```python
from build123d import *

# Parameters (mm, degrees)
PAD_DEPTH          = 38
POCKET_DEPTH       = 32
SKETCH002_R        = 6.25
POCKET001_DEPTH    = 6
CHAMFER_SIZE       = 1
SKETCH003_R        = 1.6
SKETCH003_R_2      = 3
POCKET002_DEPTH    = 7
SKETCH004_R        = 6.5
POCKET003_DEPTH    = 3
SKETCH005_R        = 1.45
POCKET004_DEPTH    = 5
POLARPATTERN_COUNT = 6
SKETCH006_R        = 3
SKETCH006_R_2      = 1.6
PAD001_DEPTH       = 1.5


with BuildPart() as part:
    # Sketch → Pad (new body)
    with BuildSketch(Plane.XY):
        with BuildLine():
            ThreePointArc((-41.5784274686, 27.7711067341), (32.1393804843, -38.3022221559), (-20.1291830613, 45.7691598053))
            Line((-41.5784274686, 27.7711067341), (-20.1291830613, 45.7691598053))
        make_face()
    extrude(amount=PAD_DEPTH)

    # Sketch001 → Pocket (cut)
    with BuildSketch(Plane.XY.offset(38)):
        with BuildLine():
            ThreePointArc((-41.314902238, 15.1353511047), (28.2826548262, -33.7059554972), (-7.7311536284, 43.3154621766))
            Line((-21.2649980047, 40.8998760372), (-7.7311536284, 43.3154621766))
            Line((-36.5858868671, 28.0441238435), (-21.2649980047, 40.8998760372))
            Line((-36.5858868671, 28.0441238435), (-41.314902238, 15.1353511047))
        make_face()
    extrude(amount=-POCKET_DEPTH, mode=Mode.SUBTRACT)

    # Sketch002 (on Face2 of Pocket) → Pocket001 (cut)
    with BuildSketch(Plane(origin=(-30.853805265, 36.7701332697, 0), x_dir=(-0.7660444431, -0.6427876097, 0), z_dir=(-0.6427876097, 0.7660444431, 0))):
        with Locations((0, 16)):
            Circle(SKETCH002_R)
    extrude(amount=-POCKET001_DEPTH, mode=Mode.SUBTRACT)

    # Chamfer
    chamfer_edges = [part.edges().sort_by_distance(p)[0] for p in [
        (32.13938, -38.302222, 0),
    ]]
    chamfer(chamfer_edges, length=CHAMFER_SIZE)

    # Sketch003 → Pocket002 (cut)
    with BuildSketch(Plane.XY.offset(6)):
        with Locations((-33.78, 19.5)):
            Circle(SKETCH003_R)
        with Locations((33.78, 19.5)):
            Circle(SKETCH003_R)
        with Locations((0, -39)):
            Circle(SKETCH003_R)
        with Locations((-25.5, 0)):
            Circle(SKETCH003_R_2)
        with Locations((25.5, 0)):
            Circle(SKETCH003_R_2)
        Polygon((-18, -6), (18, -6), (18, -17), (2, -17), (2, -22), (-2, -22), (-2, -17), (-18, -17), align=None)
    extrude(amount=-POCKET002_DEPTH, mode=Mode.SUBTRACT)

    # Sketch004 → Pocket003 (cut)
    with BuildSketch(Plane.XY.offset(6)):
        with Locations((-25.5, 0)):
            Circle(SKETCH004_R)
        with Locations((25.5, 0)):
            Circle(SKETCH004_R)
    extrude(amount=-POCKET003_DEPTH, mode=Mode.SUBTRACT)

    # Sketch005 (on Face4 of Pocket003) → Pocket004 (cut)
    with BuildSketch(Plane.XY.offset(38)):
        with Locations((0, 47)):
            Circle(SKETCH005_R)
    pocket004 = extrude(amount=-POCKET004_DEPTH, mode=Mode.SUBTRACT)

    # PolarPattern: Pocket004 ×6 about axis
    polarpattern_axis = Axis((0, 0, 38), (0, 0, 1))
    for i in range(1, POLARPATTERN_COUNT):
        add(pocket004.rotate(polarpattern_axis, i * 360 / POLARPATTERN_COUNT), mode=Mode.SUBTRACT)

    # Sketch006 (on Face34 of PolarPattern) → Pad001 (join)
    with BuildSketch(Plane.XY.offset(6)):
        with Locations((-33.78, 19.5)):
            Circle(SKETCH006_R)
        with Locations((-33.78, 19.5)):
            Circle(SKETCH006_R_2, mode=Mode.SUBTRACT)
        with Locations((33.78, 19.5)):
            Circle(SKETCH006_R)
        with Locations((33.78, 19.5)):
            Circle(SKETCH006_R_2, mode=Mode.SUBTRACT)
        with Locations((0, -39)):
            Circle(SKETCH006_R)
        with Locations((0, -39)):
            Circle(SKETCH006_R_2, mode=Mode.SUBTRACT)
    extrude(amount=PAD001_DEPTH)


solid = part.part
```
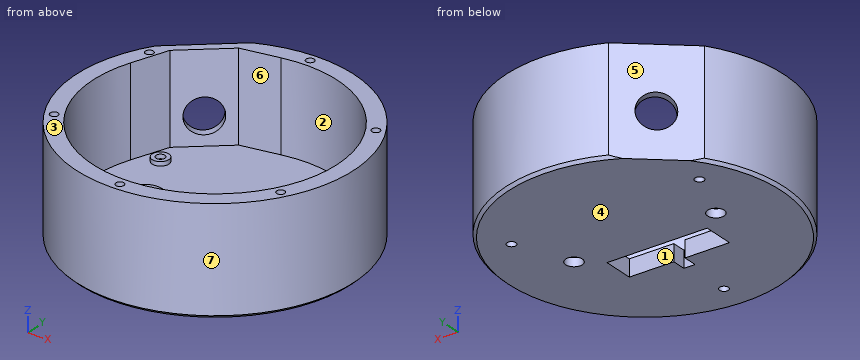
Verification items for the finished model (mm, model axes). Face numbers are marked on the shaded views. A direction names the side the tool comes from. Round coordinates to 2 decimals unless told otherwise and drop trailing zeros. Order: outer loops, then holes, each group sorted by start corner. A loop starts at its lowest first (then second) coordinate and runs counter-clockwise, first axis right, second up.
1) Draft check along Y on the marked faces 4, 5, 6 and 7. Enter one of: +Y half, -Y half, draft (parallel to the pull), parting line (faces both ways), or undercut.
Geometry says:
face 4: draft
face 5: +Y half
face 6: undercut
face 7: parting line
2) Depth check by flat-ended pin: pin 1 (1.2 mm diameter, centred on x = -1, z = 3, fed in from +Y); pin 2 (5 mm diameter, centred on x = 31.5, z = 27, fed in from -Y); pin 3 (3 mm diameter, centred on x = -12.5, z = 3.5, fed in from +Y) (3 decimals). Enter the tip coordinate at first touch or a pass-through.
Geometry says:
pin 1: stops at y = 50
pin 2: stops at y = -40.73
pin 3: stops at y = 48.775
3) Cross-section at B-B, the plane z = 35. Record the cut outline in (x, y) (3 decimals).
Geometry says:
outline: (-41.578, 27.771) arc R50 ccw (long way) to (-20.129, 45.769) - close; hole circle Ø2.9 at (-40.703, -23.5); hole circle Ø2.9 at (-40.703, 23.5); hole (-41.315, 15.135) arc R44 ccw (long way) to (-7.731, 43.315) - (-21.265, 40.9) - (-36.586, 28.044) - close; hole circle Ø2.9 at (0, -47); hole circle Ø2.9 at (0, 47); hole circle Ø2.9 at (40.703, -23.5); hole circle Ø2.9 at (40.703, 23.5)
4) Material ranges on line 1 (X direction, y = -23, z = 35); line 2 (Z direction, x = -19, y = 10.5); line 3 (Y direction, x = -8, z = 36), recorded low to high.
Geometry says:
line 1: x = -44.4 to -42.06, -39.34 to -37.51, 37.51 to 39.34, 42.06 to 44.4
line 2: z = 0 to 6
line 3: y = -49.36 to -43.27, 43.27 to 49.36
5) Cross-section at D-D, the plane z = 14. Record the cut outline in (x, y) (3 decimals), plus the area to 3 significant figures.
Geometry says:
outline: (-41.578, 27.771) arc R50 ccw (long way) to (-20.129, 45.769) - (-26.318, 40.576) - (-24.389, 38.278) - (-21.265, 40.9) - (-7.731, 43.315) arc R44 cw (long way) to (-41.315, 15.135) - (-36.586, 28.044) - (-33.461, 30.666) - (-35.39, 32.964) - close
area: 1,650 mm2
6) Cross-section at C-C, the plane z = 25.5. Record the cut outline in (x, y) (3 decimals).
Geometry says:
outline: (-41.578, 27.771) arc R50 ccw (long way) to (-20.129, 45.769) - close; hole (-41.315, 15.135) arc R44 ccw (long way) to (-7.731, 43.315) - (-21.265, 40.9) - (-36.586, 28.044) - close
7) Cross-section at A-A, the plane y = 0. Record the cut outline in (x, z).
Geometry says:
outline: (-50, 1) - (-49, 0) - (-28.5, 0) - (-28.5, 3) - (-32, 3) - (-32, 6) - (-44, 6) - (-44, 38) - (-50, 38) - close; (-22.5, 0) - (22.5, 0) - (22.5, 3) - (19, 3) - (19, 6) - (-19, 6) - (-19, 3) - (-22.5, 3) - close; (28.5, 0) - (49, 0) - (50, 1) - (50, 38) - (44, 38) - (44, 6) - (32, 6) - (32, 3) - (28.5, 3) - close
8) Tool access check on the marked faces 1, 2 and 3. Record the directions out of +Z, -Z, +X, -X, +Y, -Y that give a thin tool (end or side, any length) a straight path to the whole face; none if there is none.
Geometry says:
face 1: +Z, -Z
face 2: +Z
face 3: +Z, +X, -X, +Y, -Y
